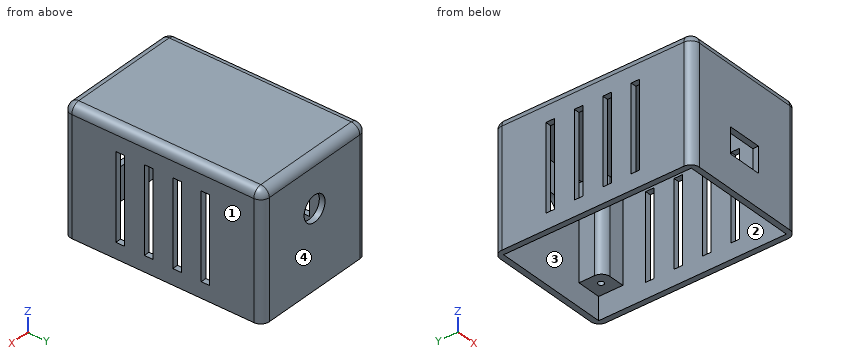
from build123d import *

# Parameters (mm, degrees)
CYLINDER_R        = 1
CYLINDER_DEPTH    = 32
BOX002_W          = 10
BOX002_H          = 10
BOX002_DEPTH      = 33
FILLET_R          = 3
BOX003_W          = 12
BOX003_H          = 20
BOX003_DEPTH      = 9
CYLINDER001_R     = 4.5
CYLINDER001_DEPTH = 10
BOX004_W          = 60
BOX004_H          = 3
BOX004_DEPTH      = 30
ARRAY_Y_COUNT     = 4
ARRAY_Y_PITCH     = 10
BOX_W             = 41
BOX_H             = 66
BOX_DEPTH         = 44
BOX001_W          = 45
BOX001_H          = 70
BOX001_DEPTH      = 44
FILLET001_R       = 3


with BuildPart() as cylinder:
    # Cylinder → Cylinder (new body)
    with BuildSketch(Plane(origin=(4, 6, 2), x_dir=(1, 0, 0), z_dir=(0, 0, 1))):
        Circle(CYLINDER_R)
    extrude(amount=CYLINDER_DEPTH)


with BuildPart() as fillet_body:
    # Box002 → Box002 (new body)
    with BuildSketch(Plane.XY.offset(2)):
        with Locations((5, 5)):
            Rectangle(BOX002_W, BOX002_H)
    extrude(amount=BOX002_DEPTH)

    # Cut: cut Cylinder
    add(cylinder.part, mode=Mode.SUBTRACT)


with BuildPart() as fillet_body_1:
    # Cut placement: moved
    add(fillet_body.part.moved(Location((12, -2, 0))))

    # Fillet
    fillet_edges = [fillet_body_1.edges().sort_by_distance(p)[0] for p in [
        (12, 8, 18.5),
        (22, -2, 18.5),
    ]]
    fillet(fillet_edges, radius=FILLET_R)


with BuildPart() as part_mirroring:
    # Part__Mirroring: instance of Fillet body
    add(fillet_body_1.part.mirror(Plane(origin=(0, 0, 0), x_dir=(0, -1, 0), z_dir=(1, 0, 0))))


with BuildPart() as part_mirroring001:
    # Part__Mirroring001: instance of Part__Mirroring
    add(part_mirroring.part.mirror(Plane(origin=(0, 32.5, 0), x_dir=(1, 0, 0), z_dir=(0, 1, 0))))


with BuildPart() as part_mirroring002:
    # Part__Mirroring002: instance of Part__Mirroring001
    add(part_mirroring001.part.mirror(Plane(origin=(0, 0, 0), x_dir=(0, -1, 0), z_dir=(1, 0, 0))))


with BuildPart() as usb_hole_cube:
    # Box003 → Box003 (new body)
    with BuildSketch(Plane(origin=(-6, -8, 5.5), x_dir=(1, 0, 0), z_dir=(0, 0, 1))):
        with Locations((6, 10)):
            Rectangle(BOX003_W, BOX003_H)
    extrude(amount=BOX003_DEPTH)


with BuildPart() as wires_hole:
    # Cylinder001 → Cylinder001 (new body)
    with BuildSketch(Plane(origin=(0, 73, 21), x_dir=(1, 0, 0), z_dir=(0, -1, 0))):
        Circle(CYLINDER001_R)
    extrude(amount=CYLINDER001_DEPTH)


with BuildPart() as array:
    # Box004 → Box004 (new body)
    with BuildSketch(Plane(origin=(-31, 16, -0.5), x_dir=(1, 0, 0), z_dir=(0, 0, 1))):
        with Locations((30, 1.5)):
            Rectangle(BOX004_W, BOX004_H)
    extrude(amount=BOX004_DEPTH)

    # Array Y: Array ×4


with BuildPart() as array_1:
    add(array.part)
    with Locations(*[(0, i * ARRAY_Y_PITCH, 0) for i in range(1, ARRAY_Y_COUNT)]):
        add(array.part)


with BuildPart() as fusion:
    # Box → Box (new body)
    with BuildSketch(Plane(origin=(-20.5, -0.5, -8), x_dir=(1, 0, 0), z_dir=(0, 0, 1))):
        with Locations((20.5, 33)):
            Rectangle(BOX_W, BOX_H)
    extrude(amount=BOX_DEPTH)

    # Fusion: union usb hole cube, wires hole, Array
    add(usb_hole_cube.part)
    add(wires_hole.part)
    add(array_1.part)


with BuildPart() as fillet001:
    # Box001 → Box001 (new body)
    with BuildSketch(Plane(origin=(-22.5, -2.5, -6), x_dir=(1, 0, 0), z_dir=(0, 0, 1))):
        with Locations((22.5, 35)):
            Rectangle(BOX001_W, BOX001_H)
    extrude(amount=BOX001_DEPTH)

    # Cut001: cut Fusion
    add(fusion.part, mode=Mode.SUBTRACT)

    # Fusion001: union Part__Mirroring002
    add(part_mirroring002.part)

    # Fillet001
    fillet001_edges = [fillet001.edges().sort_by_distance(p)[0] for p in [
        (-22.5, -2.5, 16),
        (-22.5, 32.5, 38),
        (-22.5, 67.5, 16),
        (22.5, -2.5, 16),
        (0, -2.5, 38),
        (0, 67.5, 38),
        (22.5, 32.5, 38),
        (22.5, 67.5, 16),
    ]]
    fillet(fillet001_edges, radius=FILLET001_R)


solid = fillet001.part
Can you work these out from the model? Positions are in its coordinate system, mm. Face numbers are marked on the shaded views. Give positions to 0.01 mm unless a question says otherwise; leave off trailing zeros. Loops run counter-clockwise (first coordinate to the right, second up) from the corner with the lowest first, then second, coordinate; pieces in that order, holes last. Notation, with made-up numbers: (81, -23) -> (91, -23) arc R15 cw to (91, -11) -> close; hole circle Ø2 at (-25, -2.75). An arc over 180 degrees is marked (long way). Return JSON: item names as keys, results as strings.
Q1. I want a section at C-C, the plane y = 40. List the corners of the cut face in (x, z) for me, then the cut area to 3 significant figures.
Checks:
{"outline": "(-22.5, -6) -> (-20.5, -6) -> (-20.5, 36) -> (20.5, 36) -> (20.5, -6) -> (22.5, -6) -> (22.5, 35) arc R3 ccw to (19.5, 38) -> (-19.5, 38) arc R3 ccw to (-22.5, 35) -> close", "area": "254 mm2"}
Q2. I need wall thicknesses on probe 1 along Y at (x, z) = (16, 16.5); probe 2 along X at (y, z) = (61, 9); probe 3 along Y at (x, z) = (18.5, 34.5). Which ranges of each line are inside material? Lowest first, please.
Checks:
{"probe 1": "y = -2.5 to -0.5, 57 to 60, 62 to 67.5", "probe 2": "x = -22.5 to -20.5, 12 to 15, 17 to 22.5", "probe 3": "y = -2.5 to -0.5, 57 to 67.5"}
Q3. We'd pull the mould along Y, two halves only. Please class the marked faces 1, 2, 3 and 4: released by +Y, released by -Y, zero draft, split by the parting line, or undercut.
Checks:
{"face 1": "zero draft", "face 2": "undercut", "face 3": "undercut", "face 4": "released by +Y"}
Q4. I want a section at A-A, the plane x = 0. List the corners of the cut face in (y, z) for me.
Checks:
{"outline": "(-2.5, -6) -> (-0.5, -6) -> (-0.5, 5.5) -> (-2.5, 5.5) -> close; (-2.5, 14.5) -> (-0.5, 14.5) -> (-0.5, 36) -> (65.5, 36) -> (65.5, 25.5) -> (67.5, 25.5) -> (67.5, 35) arc R3 ccw to (64.5, 38) -> (0.5, 38) arc R3 ccw to (-2.5, 35) -> close; (65.5, -6) -> (67.5, -6) -> (67.5, 16.5) -> (65.5, 16.5) -> close"}
Q5. For pin 1 Ø1 at (x, y) = (21.5, 28) entering from +Z; pin 2 Ø1.5 at (x, y) = (-17.5, 49) entering from -Z; pin 3 Ø1 at (x, z) = (-22, 12) entering from +Y, each with a flat end and sliding along its axis, tell me the tip position at first contact or that it passes through.
Checks:
{"pin 1": "stops at z = 37.6", "pin 2": "stops at z = 36", "pin 3": "stops at y = 66.74"}
Q6. I want a section at B-B, the plane z = 8.5. Count the separate pieces of the cut face and the enclosed holes in it, then the cut area to 3 significant figures.
Checks:
{"separate pieces": "9", "enclosed holes": "1", "area": "431 mm2"}
Q7. I want a section at D-D, the plane x = 16. List the corners of the cut face in (y, z) for me.
Checks:
{"outline": "(-2.5, -6) -> (-0.5, -6) -> (-0.5, 36) -> (65.5, 36) -> (65.5, 35) -> (57, 35) -> (57, 2) -> (60, 2) -> (60, 34) -> (62, 34) -> (62, 2) -> (65.5, 2) -> (65.5, -6) -> (67.5, -6) -> (67.5, 35) arc R3 ccw to (64.5, 38) -> (0.5, 38) arc R3 ccw to (-2.5, 35) -> close"}
